```python
from build123d import *

# Parameters (mm, degrees)
SKETCH_1_R      = 2
EXTRUDE_1_DEPTH = 8
EXTRUDE_START   = -12
SKETCH_3_R      = 2
EXTRUDE_2_DEPTH = 12


with BuildPart() as part:
    # ｽｹｯﾁ1 → ﾎﾞｽ - 押し出し1 (new body)
    with BuildSketch(Plane(origin=(0, 0, 0), x_dir=(1, 0, 0), z_dir=(0, 1, 0))):
        with Locations(Location((0, 0, 0), (0, 0, 270))):
            Circle(SKETCH_1_R)
    extrude(amount=EXTRUDE_1_DEPTH)

    # ｽｹｯﾁ3 → ﾎﾞｽ - 押し出し2 (add)
    with BuildSketch(Plane(origin=(0, 8, 0), x_dir=(1, 0, 0), z_dir=(0, 1, 0)).offset(EXTRUDE_START)):
        with Locations(Location((0, 0, 0), (0, 0, 270))):
            Circle(SKETCH_3_R)
    extrude(amount=EXTRUDE_2_DEPTH)

    # ｽｹｯﾁ4 → ｶｯﾄ - 回転1 (revolve, cut)
    with BuildSketch(Plane(origin=(0, 0, 0), x_dir=(0, 0, -1), z_dir=(1, 0, 0)), mode=Mode.PRIVATE) as cut_revolve_1_sk:
        Polygon((1.823673019, -4), (2, -3), (2, -4), align=None)
    revolve(cut_revolve_1_sk.sketch.rotate(Axis((0, 0, 0), (0, -1, 0)), 180), axis=Axis((0, 0, 0), (0, -1, 0)), mode=Mode.SUBTRACT)


solid = part.part
```
The model under review builds one solid part; all positions refer to its coordinate system, in mm. Give positions to 0.01 mm unless a question says otherwise; leave off trailing zeros. Write each loop counter-clockwise with the first axis right and the second up, starting at its lowest first coordinate (ties: lowest second). Pieces come first, ordered by that corner, then holes. Notation, with made-up numbers: M 40,69.5 L 61,69.5 A18 ccw 61,76.5 Z; hole C 25,-7.75 d4. An arc over 180 degrees is marked long. Answer in a Markdown table with one row per item.
Item 1: For line 1 along X through (y, z) = (3, -1.75); line 2 along Z through (x, y) = (-1, 3.5); line 3 along X through (y, z) = (3, -0.95), list the stretches that pass through material, from the lowest coordinate up.
Check sheet entries:
| item | result |
|---|---|
| line 1 | -0.97 to 0.97 |
| line 2 | -1.73 to 1.73 |
| line 3 | -1.76 to 1.76 |
Item 2: For P1, Ø1.5, axis at y = 0, z = 1, coming from the -X side; P2, Ø1.5, axis at x = -1, y = 3, coming from the -Z side, all flat-tipped, find the tip position at first contact; note any pin that passes through.
Check sheet entries:
| item | result |
|---|---|
| P1 | x = -1.98 |
| P2 | z = -1.98 |
Item 3: Add section A-A on y = 6.25. Give the boundary of the cut face in (x, z), plus the area to 3 significant figures.
Check sheet entries:
| item | result |
|---|---|
| outline | C 0,0 d4 |
| area | 12.6 mm2 |
